Here's the drawing with two shaded views (mm, measured from the low corner). I have some questions. A direction names the side the tool comes from. Give positions to 0.01 mm unless a question says otherwise; leave off trailing zeros. Write each loop counter-clockwise with the first axis right and the second up, starting at its lowest first coordinate (ties: lowest second). Pieces come first, ordered by that corner, then holes. Notation, with made-up numbers: (19, 38.5) -> (69, 38.5) arc R19 cw to (69, 64.5) -> close; hole circle Ø2 at (8.5, 83). An arc over 180 degrees is marked (long way). One line per question, with ' | ' between items.
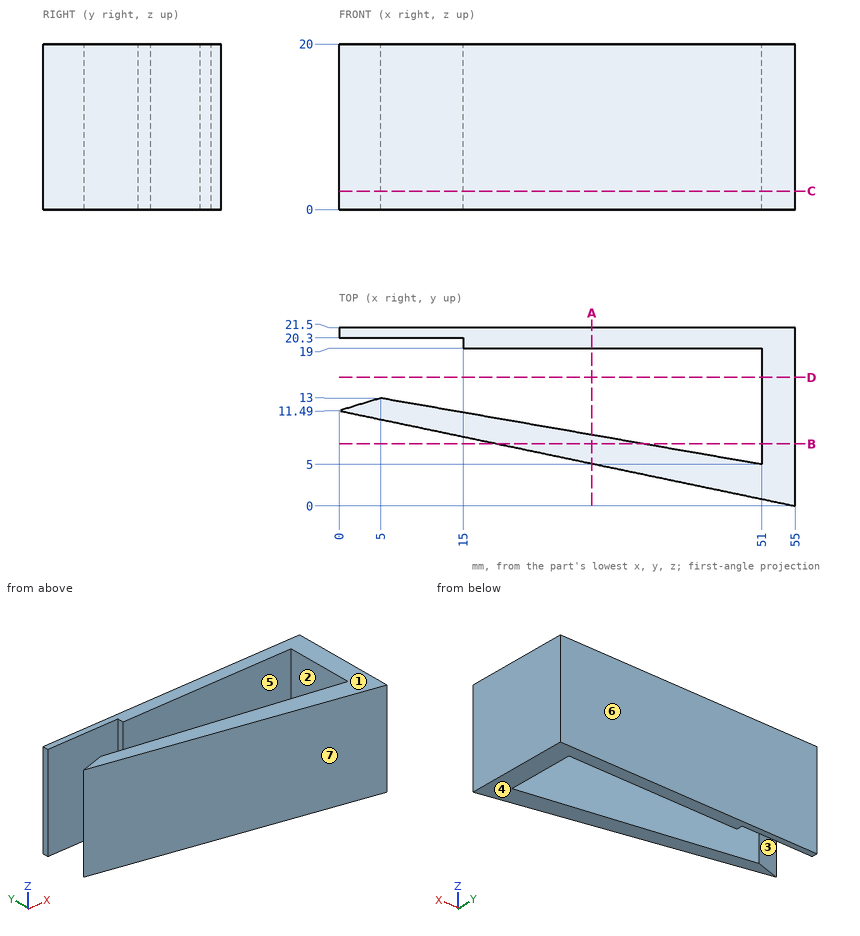
Q1. Imagine slicing it at A-A on x = 30.5. Please give me the cut outline in (y, z) (1 decimal), and give its area (3 significant figures).
Answer below:
outline: (5.1, 0) -> (8.6, 0) -> (8.6, 20) -> (5.1, 20) -> close; (19, 0) -> (21.5, 0) -> (21.5, 20) -> (19, 20) -> close | area: 119 mm^2
Q2. Imagine slicing it at D-D on y = 15.5. Please give me the cut outline in (x, z).
Answer below:
outline: (51, 0) -> (55, 0) -> (55, 20) -> (51, 20) -> close
Q3. Imagine slicing it at B-B on y = 7.5. Please give me the cut outline in (x, z) (1 decimal).
Answer below:
outline: (19.1, 0) -> (36.6, 0) -> (36.6, 20) -> (19.1, 20) -> close; (51, 0) -> (55, 0) -> (55, 20) -> (51, 20) -> close
Q4. On a 3-axis mill with a long thin cutter (end or side, diameter ignored), from which of +Z, -Z, +X, -X, +Y, -Y can I reach the whole of each face in a straight line? I mean the marked faces 1, 2 and 3. Say none if no direction works.
Answer below:
face 1: +Z, +X, -X, +Y, -Y | face 2: +Z, -Z | face 3: +Z, -Z, -X
Q5. Imagine slicing it at C-C on z = 2.25. Please give me the cut outline in (x, y), and give its area (3 significant figures).
Answer below:
outline: (0, 11.49) -> (55, 0) -> (55, 21.5) -> (0, 21.5) -> (0, 20.3) -> (15, 20.3) -> (15, 19) -> (51, 19) -> (51, 5) -> (5, 13) -> close | area: 353 mm^2
Q6. If we mould it in two halves opening along Y, with no side actions, what happens to the marked faces 4, 5, 6 and 7? For each: +Y half, -Y half, draft (parallel to the pull), parting line (faces both ways), or undercut.
Answer below:
face 4: draft | face 5: undercut | face 6: +Y half | face 7: -Y half
Q7. Will these pins go through, and if not, where does the flat tip stop? pin 1 (1 mm diameter, centred on y = 19.5, z = 7, fed in from -X); pin 2 (4.5 mm diameter, centred on x = 7, z = 13, fed in from -Y); pin 3 (8 mm diameter, centred on x = 39.5, z = 10.5, fed in from -Y).
Answer below:
pin 1: stops at x = 15 | pin 2: stops at y = 9.56 | pin 3: stops at y = 2.4
Q8. If I drill on line 1 along X through (y, z) = (20, 4); line 2 along X through (y, z) = (18.75, 1.5); line 3 along Y through (x, z) = (8, 14.75), over which ranges is the centre line in solid material (lowest first)?
Answer below:
line 1: x = 15 to 55 | line 2: x = 51 to 55 | line 3: y = 9.82 to 12.48, 20.3 to 21.5
